Build history of the part. All positions in model axes, mm. A direction names the side the tool comes from. Coordinates: 2 decimals unless noted, no trailing zeros. Loops run counter-clockwise (first coordinate to the right, second up) from the corner with the lowest first, then second, coordinate; pieces in that order, holes last.
(1) Wall check: L1, parallel to Z at x = -176, y = 82; L2, parallel to Y at x = -176.4, z = 232.5; L3, parallel to Y at x = -176, z = 232. Give the ranges that are in metal, low to high.
(2) Flat gauge pins, fed straight in: P1, Ø10, axis at x = -39.5, z = -143, coming from the -Y side; P2, Ø6, axis at y = 28, z = 230.5, coming from the +X side; P3, Ø10, axis at x = -135, y = 23.5, coming from the +Z side; P4, Ø2, axis at x = 46.5, y = 21.5, coming from the -Z side. Where does each tip first touch, or does it go through?
(3) Slice it at B-B (x = 83). Give the cut face in (y, z).
(4) Tool access for faces 1 (the face through (-177.5, 45, -3)), 2 (the face through (-175.5, 45, -231)), 3 (the face through (-175.5, 45, 231)): list every direction of +Z, -Z, +X, -X, +Y, -Y with a clear straight run to the whole face (end or side of a thin tool).
(5) Slice it at A-A (y = 20). Give the cut face in (x, z), and give its area (3 significant figures).
from build123d import *

# Parameters (mm, degrees)
CROQUIS1_W              = 355
CROQUIS1_H              = 442
SALIENTE_EXTRUIR1_DEPTH = 88
CROQUIS2_W              = 482
CROQUIS2_H              = 88
CROQUIS2_R              = 2.5
SALIENTE_EXTRUIR2_DEPTH = 2


with BuildPart() as part:
    # Croquis1 → Saliente-Extruir1 (new body)
    with BuildSketch(Plane(origin=(0, 0, 0), x_dir=(1, 0, 0), z_dir=(0, 1, 0))):
        Rectangle(CROQUIS1_W, CROQUIS1_H)
    extrude(amount=SALIENTE_EXTRUIR1_DEPTH)

    # Croquis2 → Saliente-Extruir2 (add)
    with BuildSketch(Plane.ZY.offset(177.5)):
        with Locations((0, 44)):
            Rectangle(CROQUIS2_W, CROQUIS2_H)
        with Locations((232.5, 82.1)):
            Circle(CROQUIS2_R, mode=Mode.SUBTRACT)
        with Locations((232.5, 5.9)):
            Circle(CROQUIS2_R, mode=Mode.SUBTRACT)
        with Locations((-232.5, 5.9)):
            Circle(CROQUIS2_R, mode=Mode.SUBTRACT)
        with Locations((-232.5, 82.1)):
            Circle(CROQUIS2_R, mode=Mode.SUBTRACT)
    extrude(amount=-SALIENTE_EXTRUIR2_DEPTH)


solid = part.part
Response values:
1. L1: z = -241 to -235, -230 to 230, 235 to 241
1. L2: y = 0 to 3.4, 8.4 to 79.6, 84.6 to 88
1. L3: y = 0 to 3.45, 8.35 to 79.65, 84.55 to 88
2. P1: stops at y = 0
2. P2: stops at x = -175.5
2. P3: stops at z = 221
2. P4: stops at z = -221
3. outline: (0, -221) - (88, -221) - (88, 221) - (0, 221) - close
4. face 1: +Z, -Z, -X, +Y, -Y
4. face 2: -Z, +X, +Y, -Y
4. face 3: +Z, +X, +Y, -Y
5. outline: (-177.5, -241) - (-175.5, -241) - (-175.5, -221) - (177.5, -221) - (177.5, 221) - (-175.5, 221) - (-175.5, 241) - (-177.5, 241) - close
5. area: 157,000 mm2
